Autodesk Inventor part; units mm, degrees
ref_plane "YZ Plane" through (0, 0, 0) normal (1, 0, 0) x (0, 1, 0)
ref_plane "XZ Plane" through (0, 0, 0) normal (0, 1, 0) x (-1, 0, 0)
ref_plane "XY Plane" through (0, 0, 0) normal (0, 0, 1) x (1, 0, 0)
sketch "Sketch1" plane through (0, 0, 0) normal (0, 0, 1) x (1, 0, 0)
  circle A0 centre (12.7, -12.7) radius 1.5875
  line L0 (0, 0) -> (0, -14.9496)
  line L1 (0, 0) -> (27.0799, 0)
  circle A1 centre (25.4, -12.7) radius 1.5875
  circle A2 centre (38.1, -12.7) radius 1.5875
  circle A3 centre (50.8, -12.7) radius 1.5875
  circle A4 centre (63.5, -12.7) radius 1.5875
  circle A5 centre (12.7, -25.4) radius 1.5875
  circle A6 centre (12.7, -38.1) radius 1.5875
  circle A7 centre (12.7, -50.8) radius 1.5875
  circle A8 centre (12.7, -63.5) radius 1.5875
  line L2 (27.0799, 0) -> (66.675, 0)
  line L3 (69.85, -3.175) -> (69.85, -22.225)
  line L4 (0, -14.9496) -> (0, -66.675)
  line L5 (3.175, -69.85) -> (22.225, -69.85)
  line L6 (66.675, -25.4) -> (33.02, -25.4)
  line L7 (25.4, -33.02) -> (25.4, -66.675)
  arc A9 (33.02, -25.4) -> (25.4, -33.02) centre (33.02, -33.02) ccw
  line L8 (66.675, 0) -> (69.85, -3.175)
  line L9 (66.675, -25.4) -> (69.85, -22.225)
  line L10 (0, -66.675) -> (3.175, -69.85)
  line L11 (22.225, -69.85) -> (25.4, -66.675)
  line L12 (0, -1.5875) -> (1.5875, 0)
  point P0 (69.85, 0)
  point P1 (69.85, -25.4)
  point P2 (69.85, -12.7)
  point P3 (0, -69.85)
  point P4 (25.4, -69.85)
  dimension "d0" = 3.175
  dimension "d1" = 12.7
  dimension "d2" = 12.7
  dimension "d5" = 12.7
  dimension "d12" = 12.7
  dimension "d17" = 6.35
  dimension "d18" = 25.4
  dimension "d19" = 6.35
  dimension "d20" = 25.4
  dimension "d21" = 7.62
  dimension "d22" = 3.175
  dimension "d23" = 3.175
  dimension "d24" = 3.175
  dimension "d25" = 3.175
  dimension "d26" = 3.175
  dimension "d27" = 3.175
  dimension "d28" = 3.175
  dimension "d29" = 3.175
extrude "Extrusion1" add sketch "Sketch1" along normal blind 3.175 contours L12 L1 L2 L8 L3 L9 L6 A9 L7 L11 L5 L10 L4 L0
properties part number "L-Bracket"
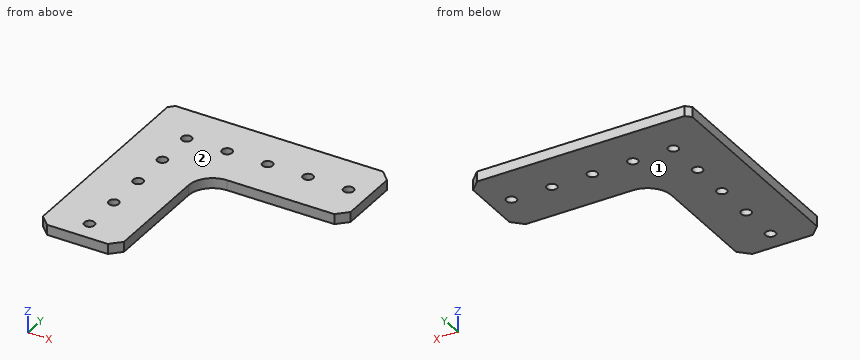
Could you check a few things on this model? Use its own coordinates, in mm. Face numbers are marked on the shaded views. Coordinates: 2 decimals unless noted, no trailing zeros. Loops run counter-clockwise (first coordinate to the right, second up) from the corner with the lowest first, then second, coordinate; pieces in that order, holes last.
1. Imagine slicing it at C-C (y = -63.5). Please give me the cut outline in (x, z) (1 decimal), and give its area (3 significant figures).
2. Imagine slicing it at D-D (x = 63.5). Please give me the cut outline in (y, z) (1 decimal), and give its area (3 significant figures).
3. I need wall thicknesses on L1, parallel to Y at x = 12.7, z = 1.75; L2, parallel to Y at x = 50.8, z = 2.15; L3, parallel to Y at x = 39, z = 2.8. Which ranges of each line are inside material? Lowest first, please.
4. We'd pull the mould along Z, two halves only. Please class the marked faces 1 and 2: released by +Z, released by -Z, zero draft, split by the parting line, or undercut.
5. For P1, Ø1.6, axis at y = -51, z = 2, coming from the +X side; P2, Ø3, axis at x = 38.1, y = -12.7, coming from the -Z side, each with a flat end and sliding along its axis, tell me the tip position at first contact or that it passes through.
6. Imagine slicing it at A-A (x = 12.7). Give the number of separate pieces and of enclosed holes in the cut face, and give its area (3 significant figures).
Computed values:
1. outline: (0, 0) - (11.1, 0) - (11.1, 3.2) - (0, 3.2) - close; (14.3, 0) - (25.4, 0) - (25.4, 3.2) - (14.3, 3.2) - close
1. area: 70.6 mm2
2. outline: (-25.4, 0) - (-14.3, 0) - (-14.3, 3.2) - (-25.4, 3.2) - close; (-11.1, 0) - (0, 0) - (0, 3.2) - (-11.1, 3.2) - close
2. area: 70.6 mm2
3. L1: y = -69.85 to -65.09, -61.91 to -52.39, -49.21 to -39.69, -36.51 to -26.99, -23.81 to -14.29, -11.11 to 0
3. L2: y = -25.4 to -14.29, -11.11 to 0
3. L3: y = -25.4 to -14.01, -11.39 to 0
4. face 1: released by -Z
4. face 2: released by +Z
5. P1: stops at x = 25.4
5. P2: passes through
6. separate pieces: 6
6. enclosed holes: 0
6. area: 171 mm2
